The model under review builds one solid part; all positions refer to its coordinate system, in mm. A direction names the side the tool comes from. Coordinates: 2 decimals unless noted, no trailing zeros. Order: outer loops, then holes, each group sorted by start corner. A loop starts at its lowest first (then second) coordinate and runs counter-clockwise, first axis right, second up. Notation, with made-up numbers: (25, 82) -> (56, 82) arc R26 ccw to (56, 98) -> close; hole circle Ø9 at (20.5, 33.25). An arc over 180 degrees is marked (long way). Put each result on its own line as item: value.
from build123d import *

# Parameters (mm, degrees)
F1_DEPTH  = 20
F2_DEPTH  = 20
F3_DEPTH  = 1
F4_DEPTH  = 2
F5_R      = 5
F6_R      = 3.125
F7_DEPTH  = 3
F9_DEPTH  = 20
F10_DEPTH = 2
F11_DEPTH = 0.2030410289
F12_DEPTH = 0.1843461736
F13_R     = 3
F14_DEPTH = 13


with BuildPart() as f1:
    # F0 (on Top) → F1 (new body)
    with BuildSketch(Plane.XY):
        with BuildLine():
            Line((-15, -22.5), (0, -22.5))
            Line((0, -22.5), (0, -20))
            ThreePointArc((0, -20), (-10, -10), (0, 0))
            Line((0, 0), (0, 6))
            Line((0, 6), (-15, 6))
            Line((-15, 6), (-15, -22.5))
        make_face()
    extrude(amount=F1_DEPTH)

    # F0 (on Top) → F2 (join)
    with BuildSketch(Plane.XY):
        with BuildLine():
            ThreePointArc((0, -47), (-11, -36), (0, -25))
            Line((0, -25), (0, -22.5))
            Line((0, -22.5), (-15, -22.5))
            Line((-15, -22.5), (-15, -52))
            Line((-15, -52), (0, -52))
            Line((0, -52), (0, -47))
        make_face()
    extrude(amount=F2_DEPTH)

    # F3 (cut): a face of the model
    f3_faces = [f1.faces().sort_by_distance(p)[0] for p in [
        (0, 3, 10),
    ]]
    extrude(f3_faces, amount=-F3_DEPTH, mode=Mode.SUBTRACT)

    # F4 (cut): a face of the model
    f4_faces = [f1.faces().sort_by_distance(p)[0] for p in [
        (-0.5, 0, 10),
    ]]
    extrude(f4_faces, amount=-F4_DEPTH, mode=Mode.SUBTRACT)

    # F5
    f5_edges = [f1.edges().sort_by_distance(p)[0] for p in [
        (-15, -52, 10),
    ]]
    fillet(f5_edges, radius=F5_R)

    # F6 (on face) → F7 (cut)
    with BuildSketch(Plane(origin=(-15, 0, 0), x_dir=(0, -1, 0), z_dir=(-1, 0, 0))):
        Polygon((16.1327298143, 13.3499298867), (16.1760774277, 6.6500701133), (22, 3.3376803609), (27.7805749589, 6.725150382), (27.7372273456, 13.4250101555), (21.9133047732, 16.7373999079), align=None)
        with Locations((22, 10)):
            Circle(F6_R, mode=Mode.SUBTRACT)
    extrude(amount=-F7_DEPTH, mode=Mode.SUBTRACT)

    # F8 (on face) → F9 (cut, through all)
    with BuildSketch(Plane.XY.offset(20)):
        with BuildLine():
            Line((-15, 6), (-15, -3.4501256289))
            Line((-15, -3.4501256289), (-7.5563976684, -3.4501256289))
            ThreePointArc((-7.5563976684, -3.4501256289), (-4.6035839587, -1.1226684902), (-1, -0.0501256289))
            Line((-1, -0.0501256289), (-1, 6))
            Line((-1, 6), (-15, 6))
        make_face()
    extrude(amount=-F9_DEPTH, mode=Mode.SUBTRACT)

    # F10 (cut): a face of the model
    f10_faces = [f1.faces().sort_by_distance(p)[0] for p in [
        (0, -22.5, 10),
    ]]
    extrude(f10_faces, amount=-F10_DEPTH, mode=Mode.SUBTRACT)

    # F11 (cut, through all): a face of the model
    f11_faces = [f1.faces().sort_by_distance(p)[0] for p in [
        (-1, -20, 10),
    ]]
    extrude(f11_faces, amount=-F11_DEPTH, mode=Mode.SUBTRACT)

    # F12 (cut, through all): a face of the model
    f12_faces = [f1.faces().sort_by_distance(p)[0] for p in [
        (-1, -25, 10),
    ]]
    extrude(f12_faces, amount=-F12_DEPTH, mode=Mode.SUBTRACT)

    # F13
    f13_edges = [f1.edges().sort_by_distance(p)[0] for p in [
        (0, -52, 10),
    ]]
    fillet(f13_edges, radius=F13_R)

    # F14 (cut, through all): a face of the model
    f14_faces = [f1.faces().sort_by_distance(p)[0] for p in [
        (-15, -22, 10),
    ]]
    extrude(f14_faces, amount=-F14_DEPTH, mode=Mode.SUBTRACT)


solid = f1.part
Item 1: For faces 1 (the flat face through (-2, -24.3, 7.6)), 2 (the flat face through (-13.521, -19.063, 15.067)), 3 (the flat face through (-11, -27, 0)), list the 3-axis set-ups (+Z, -Z, +X, -X, +Y, -Y) from which the entire face can be reached by the end or side of a thin tool; tool diameter is ignored.
Answers below:
face 1: +Z, -Z, +X, +Y
face 2: -X
face 3: -Z, +X, -X, +Y, -Y
Item 2: For line 1 (Z direction, x = -7.25, y = -22) (3 decimals); line 2 (Y direction, x = -8.75, z = 10) (3 decimals); line 3 (Y direction, x = -8.75, z = 8), list the stretches that pass through material, from the lowest coordinate up. Write a range as from..to.
Answers below:
line 1: 0..6.875, 13.125..20
line 2: -52..-42.666, -29.334..-25.125, -18.875..-14.841, -5.159..-3.45
line 3: -52..-42.67, -29.33..-24.4, -19.6..-14.84, -5.16..-3.45
Item 3: For pin 1 Ø10 at (y, z) = (-22, 10) entering from +X; pin 2 Ø10 at (y, z) = (-37.5, 5.5) entering from +X; pin 3 Ø3 at (y, z) = (-18, 10.5) entering from -X, all flat-tipped, find the tip position at first contact; note any pin that passes through.
Answers below:
pin 1: x = -2
pin 2: x = -8.87
pin 3: x = -12
Item 4: Consider section A-A on z = 10. Write out the cut boundary in (x, y) (3 decimals), and give its area (3 significant figures).
Answers below:
outline: (-15, -47) arc R5 ccw to (-10, -52) -> (-3, -52) arc R3 ccw to (0, -49) -> (0, -47) arc R11 cw to (-2, -25.183) -> (-2, -25.125) -> (-12, -25.125) -> (-12, -27.759) -> (-15, -27.759) -> close; (-15, -16.154) -> (-12, -16.154) -> (-12, -18.875) -> (-4.608, -18.875) arc R10 cw to (-7.556, -3.45) -> (-15, -3.45) -> close
area: 286 mm^2
Item 5: Consider section D-D on x = -4.5. Write out the cut boundary in (y, z) (3 decimals), and give its area (3 significant figures).
Answers below:
outline: (-52, 0) -> (-46.037, 0) -> (-46.037, 20) -> (-52, 20) -> close; (-25.963, 0) -> (-18.93, 0) -> (-18.93, 9.415) arc R3.125 cw (long way) to (-18.93, 10.585) -> (-18.93, 20) -> (-25.963, 20) -> close
area: 229 mm^2
Item 6: Consider section B-B on x = -12.75. Write out the cut boundary in (y, z).
Answers below:
outline: (-51.18, 0) -> (-3.45, 0) -> (-3.45, 20) -> (-51.18, 20) -> close; hole (-27.78, 6.73) -> (-22, 3.34) -> (-16.18, 6.65) -> (-16.13, 13.35) -> (-21.91, 16.74) -> (-27.74, 13.43) -> close
Item 7: Mouldability with a two-part tool opening along Z and no side actions: class faces 4 (the cylindrical face through (-7.07, -24.98, 10.94)), 5 (the cylindrical face through (-14, -50, 10)), 6 (the flat face through (-11, -27, 20)) as +Z half, -Z half, draft (parallel to the pull), parting line (faces both ways), or undercut.
Answers below:
face 4: undercut
face 5: draft
face 6: +Z half
Item 8: Consider section C-C on x = -6.5. Write out the cut boundary in (y, z) (3 decimals), and give its area (3 significant figures).
Answers below:
outline: (-52, 0) -> (-44.874, 0) -> (-44.874, 20) -> (-52, 20) -> close; (-27.126, 0) -> (-17.599, 0) -> (-17.599, 20) -> (-27.126, 20) -> close; hole circle Ø6.25 at (-22, 10)
area: 302 mm^2
